from build123d import *

# Parameters (mm, degrees)
F0_R     = 13.8
F1_DEPTH = 3
F2_R     = 8.1
F3_DEPTH = 25
F2_R_2   = 11.25
F4_DEPTH = 10
F5_SIZE  = 2.99999


# Not quite as in the source:
# - a fillet or chamfer is up to 0.001 mm smaller than in the source, because OpenCascade refuses the exact size


with BuildPart() as f1:
    # F0 (on Front) → F1 (new body)
    with BuildSketch(Plane.XZ):
        Circle(F0_R)
    extrude(amount=F1_DEPTH)

    # F2 (on face) → F3 (cut)
    with BuildSketch(Plane.XZ.offset(3)):
        Circle(F2_R)
    extrude(amount=-F3_DEPTH, mode=Mode.SUBTRACT)

    # F2 (on face) → F4 (join)
    with BuildSketch(Plane.XZ.offset(3)):
        Circle(F2_R_2)
        Circle(F2_R, mode=Mode.SUBTRACT)
    extrude(amount=-F4_DEPTH)

    # F5 (size 3 in the source; OpenCascade refuses exactly that, so slightly less here)
    f5_edges = [f1.edges().sort_by_distance(p)[0] for p in [
        (-13.8, -3, 0),
    ]]
    chamfer(f5_edges, length=F5_SIZE)


solid = f1.part
Design review of the part built by this model. Coordinates are the model's own, in mm. A direction names the side the tool comes from. Round coordinates to 2 decimals unless told otherwise and drop trailing zeros. Order: outer loops, then holes, each group sorted by start corner. A loop starts at its lowest first (then second) coordinate and runs counter-clockwise, first axis right, second up.
1) Consider section C-C (y = 6). State the section outline as (x, z) points, plus the area to 3 significant figures.
The answers:
outline: circle Ø22.5 at (0, 0); hole circle Ø16.2 at (0, 0)
area: 191 mm2
2) Draft analysis for pull direction Z (two halves, no side actions). For faces 1 (the conical face through (10.44, -2.854, 3.288)), 2 (the cylindrical face through (-1.756, 1.93, -7.907)), 3 (the flat face through (-5.2, 0, -10.2)), state which applies: released by +Z, released by -Z, zero draft, split by the parting line, or undercut.
The answers:
face 1: split by the parting line
face 2: undercut
face 3: zero draft
3) Consider section D-D (y = -2). State the section outline as (x, z) points.
The answers:
outline: circle Ø23.6 at (0, 0); hole circle Ø16.2 at (0, 0)
4) For L1, parallel to Z at x = 0, y = 1; L2, parallel to X at y = 2.25, z = -3.75; L3, parallel to X at y = 3.5, z = 1.75, list the stretches that pass through material, from the lowest coordinate up.
The answers:
L1: z = -11.25 to -8.1, 8.1 to 11.25
L2: x = -10.61 to -7.18, 7.18 to 10.61
L3: x = -11.11 to -7.91, 7.91 to 11.11
5) Clearance check with flat-ended pins moving along their axes: pin 1 Ø6 at (x, y) = (-5.5, 4.5) entering from -Z; pin 2 Ø6 at (y, z) = (3.5, -3.5) entering from -X. State where each tip first meets the part, or that it passes through.
The answers:
pin 1: stops at z = -10.97
pin 2: stops at x = -11.24
6) Machinability: for faces 4 (the flat face through (-8, 7, 3)), 5 (the cylindrical face through (5.19, 3.45, -9.98)), which of the approach directions +Z, -Z, +X, -X, +Y, -Y give a long, thin tool a straight path to every point of the face, cutting with its end or side? Answer none if there is none.
The answers:
face 4: +Z, -Z, +X, -X, +Y
face 5: +Y
